Check sheet for the modelled part. Datum: model origin and axes. Units: mm. Give positions to 0.01 mm unless a question says otherwise; leave off trailing zeros. Order: outer loops, then holes, each group sorted by start corner. A loop starts at its lowest first (then second) coordinate and runs counter-clockwise, first axis right, second up. Notation, with made-up numbers: (-8, 80.5) -> (38, 80.5) arc R32 ccw to (38, 112.5) -> close; hole circle Ø5 at (76, 6.25). An arc over 180 degrees is marked (long way). Write each question's results on one line, items separated by ' | '.
from build123d import *

# Parameters (mm, degrees)
F2_R     = 30.1625
F3_DEPTH = 251.001


with BuildPart() as f1:
    # F0 (on Front) → F1 (revolve)
    with BuildSketch(Plane.XZ):
        with BuildLine():
            Line((-800, -30), (-800, 0))
            Line((-800, 0), (-806, 0))
            Line((-806, 0), (-806, -30))
            ThreePointArc((-806, -30), (-795.245431, -66.110142), (-766.486595, -90.452132))
            ThreePointArc((-766.486595, -90.452132), (-391.560123, -210.432198), (0, -251))
            Line((0, -251), (0, -245))
            ThreePointArc((0, -245), (-390.33006, -204.55964), (-764.078723, -84.956484))
            ThreePointArc((-764.078723, -84.956484), (-790.223119, -62.827402), (-800, -30))
        make_face()
    revolve(axis=Axis((0, 0, -122.5), (0, 0, -1)))

    # F2 (on Top) → F3 (cut, through all)
    with BuildSketch(Plane.XY):
        Circle(F2_R)
    extrude(amount=-F3_DEPTH, mode=Mode.SUBTRACT)


solid = f1.part
1. Section check A-A on z = -64. Record the cut outline in (x, y), then the cut area to 3 significant figures.
Verdict:
outline: circle Ø1593.14 at (0, 0); hole circle Ø1578.87 at (0, 0) | area: 35,500 mm^2
2. Mould release check, pull along Y, two halves, no side actions. Record for faces 1 (the cylindrical face through (104.93, 799.14, -15.21)), 2 (the cylindrical face through (-763.057, 240.298, -14.79)): +Y half, -Y half, draft (parallel to the pull), parting line (faces both ways), or undercut.
Verdict:
face 1: parting line | face 2: undercut
3. Gauge pin test, flat ends, axial feed: pin 1 Ø5 at (x, y) = (514, -467) entering from -Z; pin 2 Ø10 at (y, z) = (148.5, -60.5) entering from +X; pin 3 Ø8 at (x, z) = (334.5, -38.5) entering from -Y. Record the tip position at first contact, or that the pin passes through.
Verdict:
pin 1: stops at z = -121.24 | pin 2: stops at x = 787.18 | pin 3: stops at y = -734.6
4. Material ranges on probe 1 along Y at (x, z) = (0, -15.25); probe 2 along Y at (x, z) = (-277, -62.5); probe 3 along X at (y, z) = (-362, -41), recorded low to high. Write a range as from..to.
Verdict:
probe 1: y = -806..-800, 800..806 | probe 2: y = -747.79..-740.31, 740.31..747.79 | probe 3: x = -719.1..-712.27, 712.27..719.1
